from build123d import *

# Parameters (mm, degrees)
SKETCH1_R          = 114.5
BASE_FLANGE1_DEPTH = 4
SKETCH2_R          = 4.6
EXTRUDE1_DEPTH     = 4
SKETCH3_R          = 5.5
EXTRUDE2_DEPTH     = 4
CIRPATTERN1_COUNT  = 8


# Sheet-metal steps are written as plain solids
with BuildPart() as part:
    # Sketch1 → Base-Flange1 (new body)
    with BuildSketch(Plane.XY):
        with BuildLine():
            Line((269, 269), (269, 325))
            Line((269, 325), (229, 325))
            Line((229, 325), (229, 295))
            ThreePointArc((229, 295), (0, 185.967739138), (-229, 295))
            Line((-229, 295), (-229, 325))
            Line((-229, 325), (-269, 325))
            Line((-269, 325), (-269, 269))
            Line((-269, 269), (-325, 269))
            Line((-325, 269), (-325, 229))
            Line((-325, 229), (-295, 229))
            ThreePointArc((-295, 229), (-185.967739138, 0), (-295, -229))
            Line((-295, -229), (-325, -229))
            Line((-325, -229), (-325, -269))
            Line((-325, -269), (-269, -269))
            Line((-269, -269), (-269, -325))
            Line((-269, -325), (-229, -325))
            Line((-229, -325), (-229, -295))
            ThreePointArc((-229, -295), (0, -185.967739138), (229, -295))
            Line((229, -295), (229, -325))
            Line((229, -325), (269, -325))
            Line((269, -325), (269, -269))
            Line((269, -269), (325, -269))
            Line((325, -269), (325, -229))
            Line((325, -229), (295, -229))
            ThreePointArc((295, -229), (185.967739138, 0), (295, 229))
            Line((295, 229), (325, 229))
            Line((325, 229), (325, 269))
            Line((325, 269), (269, 269))
        make_face()
        Circle(SKETCH1_R, mode=Mode.SUBTRACT)
    extrude(amount=BASE_FLANGE1_DEPTH)

    # Sketch2 → Extrude1 (cut)
    with BuildSketch(Plane.XY.offset(4)):
        with Locations((249, 312.5)):
            Circle(SKETCH2_R)
        with Locations((249, 282.5)):
            Circle(SKETCH2_R)
        with Locations((282.5, 249)):
            Circle(SKETCH2_R)
        with Locations((312.5, 249)):
            Circle(SKETCH2_R)
        with Locations(Location((312.5, -249, 0), (0, 0, 180))):
            Circle(SKETCH2_R)
        with Locations(Location((282.5, -249, 0), (0, 0, 180))):
            Circle(SKETCH2_R)
        with Locations(Location((249, -282.5, 0), (0, 0, 180))):
            Circle(SKETCH2_R)
        with Locations(Location((249, -312.5, 0), (0, 0, 180))):
            Circle(SKETCH2_R)
        with Locations((-249, -312.5)):
            Circle(SKETCH2_R)
        with Locations((-249, -282.5)):
            Circle(SKETCH2_R)
        with Locations((-282.5, -249)):
            Circle(SKETCH2_R)
        with Locations((-312.5, -249)):
            Circle(SKETCH2_R)
        with Locations(Location((-312.5, 249, 0), (0, 0, 180))):
            Circle(SKETCH2_R)
        with Locations(Location((-282.5, 249, 0), (0, 0, 180))):
            Circle(SKETCH2_R)
        with Locations(Location((-249, 282.5, 0), (0, 0, 180))):
            Circle(SKETCH2_R)
        with Locations(Location((-249, 312.5, 0), (0, 0, 180))):
            Circle(SKETCH2_R)
    extrude(amount=-EXTRUDE1_DEPTH, mode=Mode.SUBTRACT)

    # Sketch3 → Extrude2 (cut)
    with BuildSketch(Plane.XY.offset(4)):
        with Locations((0, 126)):
            Circle(SKETCH3_R)
    extrude2 = extrude(amount=-EXTRUDE2_DEPTH, mode=Mode.SUBTRACT)

    # CirPattern1: Extrude2 ×8 about axis
    cirpattern1_axis = Axis((0, 0, 0), (0, 0, 1))
    for i in range(1, CIRPATTERN1_COUNT):
        add(extrude2.rotate(cirpattern1_axis, i * 360 / CIRPATTERN1_COUNT), mode=Mode.SUBTRACT)


solid = part.part
Verification items for the finished model (mm, model axes). Coordinates: 2 decimals unless noted, no trailing zeros. Write each loop counter-clockwise with the first axis right and the second up, starting at its lowest first coordinate (ties: lowest second). Pieces come first, ordered by that corner, then holes. Notation, with made-up numbers: (35.5, -16) -> (86.5, -16) arc R30 cw to (86.5, 14) -> close; hole circle Ø9 at (-14, 38.5). An arc over 180 degrees is marked (long way). One line per item, written item: value. Start each with the question number.
Q1. Cross-section at D-D on x = 164. Enter the section's corners in (y, z), and give its area (3 significant figures).
Q2. Thickness scan on L1, parallel to Y at x = -312.5, z = 1.4; L2, parallel to X at y = -3.5, z = 3.45; L3, parallel to Y at x = -282.5, z = 1.55. Record the ranges inside material, lowest first. Write a range as from..to.
Q3. Go/stop test with flat-tipped pins: P1, Ø5, axis at x = -114, y = -169, coming from the -Z side; P2, Ø2, axis at y = 306.5, z = 2, coming from the +X side; P3, Ø1.5, axis at y = -47, z = 3, coming from the +X side; P4, Ø1, axis at y = 185, z = 2.5, coming from the +X side. Record where each tip stops, or that it passes through.
Q4. Cross-section at B-B on x = -105. Enter the section's corners in (y, z).
Q5. Mould release check, pull along X, two halves, no side actions. Record for faces 1 (the cylindrical face through (-3.67, -185.99, 1.97)), 2 (the cylindrical face through (185.99, -3.67, 1.97)), 3 (the cylindrical face through (-185.99, 3.67, 1.97)): pulls with the +X half, pulls with the -X half, needs draft (parallel to the pull), parting line crosses it, or undercut.
Q6. Cross-section at A-A on y = 202.5. Enter the section's corners in (x, z), and give its area (3 significant figures).
Q7. Cross-section at C-C on z = 2.65. State how many separate pieces and enclosed holes the cut face has, and give its area (3 significant figures).
Checked values:
1. outline: (-235.76, 0) -> (235.76, 0) -> (235.76, 4) -> (-235.76, 4) -> close
1. area: 1,890 mm²
2. L1: y = -269..-253.6, -244.4..-229, 229..244.4, 253.6..269
2. L2: x = -185.99..-130.24, -121.76..-114.45, 114.45..121.76, 130.24..185.99
2. L3: y = -269..-253.6, -244.4..-218.26, 218.26..244.4, 253.6..269
3. P1: stops at z = 0
3. P2: stops at x = 269
3. P3: stops at x = 189.86
3. P4: stops at x = 251.59
4. outline: (-205.29, 0) -> (-45.66, 0) -> (-45.66, 4) -> (-205.29, 4) -> close; (45.66, 0) -> (205.29, 0) -> (205.29, 4) -> (45.66, 4) -> close
5. face 1: undercut
5. face 2: pulls with the +X half
5. face 3: pulls with the -X half
6. outline: (-266.45, 0) -> (-97.37, 0) -> (-97.37, 4) -> (-266.45, 4) -> close; (97.37, 0) -> (266.45, 0) -> (266.45, 4) -> (97.37, 4) -> close
6. area: 1,350 mm²
7. separate pieces: 1
7. enclosed holes: 25
7. area: 173,000 mm²
